Autodesk Inventor part; units mm, degrees
ref_plane "YZ Plane" through (0, 0, 0) normal (1, 0, 0) x (0, 1, 0)
ref_plane "XZ Plane" through (0, 0, 0) normal (0, 1, 0) x (-1, 0, 0)
ref_plane "XY Plane" through (0, 0, 0) normal (0, 0, 1) x (1, 0, 0)
sketch "Boceto1" plane through (0, 0, 0) normal (0, 0, 1) x (1, 0, 0)
  line L0 (0, 0) -> (20, 0)
  line L1 (20, 0) -> (20, 35)
  line L2 (20, 35) -> (0, 35)
  line L3 (0, 35) -> (0, 0)
  line L4 (10, 31) -> (10, 26) construction
  line L5 (8, 31) -> (8, 26)
  line L6 (12, 26) -> (12, 31)
  arc A0 (12, 31) -> (8, 31) centre (10, 31) ccw
  arc A1 (8, 26) -> (12, 26) centre (10, 26) ccw
  line L7 (10, 4) -> (10, 9) construction
  line L8 (12, 4) -> (12, 9)
  line L9 (8, 9) -> (8, 4)
  arc A2 (8, 4) -> (12, 4) centre (10, 4) ccw
  arc A3 (12, 9) -> (8, 9) centre (10, 9) ccw
  point P0 (10, 28.5)
  point P1 (10, 6.5)
  point P2 (10, 33)
  point P3 (10, 2)
  point P4 (10, 11)
  point P5 (10, 24)
  dimension "d0" = 20
  dimension "d1" = 35
  dimension "d2" = 5
  dimension "d3" = 4
  dimension "d4" = 5
  dimension "d5" = 4
  dimension "d6" = 2
  dimension "d7" = 2
  dimension "d8" = 13
extrude "Extrusión1" add sketch "Boceto1" along normal blind 2
sketch "Boceto2" plane through (0, 0, 2) normal (0, 0, 1) x (1, 0, 0)
  line L0 (8, 26) -> (8, 31)
  line L1 (12, 31) -> (12, 26)
  line L2 (8, 21.5) -> (12, 21.5)
  line L3 (12, 21.5) -> (12, 13.5)
  line L4 (12, 13.5) -> (8, 13.5)
  line L5 (8, 13.5) -> (8, 21.5)
  arc A0 (8, 26) -> (12, 26) centre (10, 26) ccw
  arc A1 (12, 9) -> (8, 9) centre (10, 9) ccw
  circle A2 centre (10, 17.5) radius 1.5
  point P0 (0, 0)
  point P1 (10, 21.5)
  point P2 (10, 24)
  point P3 (10, 13.5)
  point P4 (10, 11)
  dimension "d11" = 4
  dimension "d12" = 8
  dimension "d13" = 2.5
  dimension "d15" = 3
extrude "Extrusión2" add sketch "Boceto2" along normal blind 1
sketch "Boceto3" plane through (8, 21.5, 2) normal (0, 1, 0) x (1, 0, 0)
  line L0 (0, -1) -> (0, -6)
  line L1 (4, -1) -> (4, -6)
  arc A0 (0, -6) -> (4, -6) centre (2, -6) ccw
  circle A1 centre (2, -6) radius 1.25
  line L2 (0, -1) -> (4, -1)
  line L3 (0, -1) -> (4, -1)
  point P0 (-8, 2)
  dimension "d18" = 5
  dimension "d19" = 5
  dimension "d20" = 2
  dimension "d21" = 2.5
extrude "Extrusión3" add sketch "Boceto3" against normal blind 1
sketch "Boceto4" plane through (8, 13.5, 2) normal (0, -1, 0) x (1, 0, 0)
  line L0 (0, 0) -> (0, 6)
  line L1 (0, 1) -> (0, 6)
  line L2 (4, 0) -> (4, 1)
  line L3 (4, 1) -> (4, 6)
  line L4 (4, 1) -> (4, 6)
  arc A0 (4, 6) -> (0, 6) centre (2, 6) ccw
  circle A1 centre (2, 6) radius 1.25
  line L5 (0, 1) -> (4, 1)
  line L6 (0, 1) -> (4, 1)
  point P0 (-8, -2)
  dimension "d25" = 2.5
extrude "Extrusión4" add sketch "Boceto4" against normal blind 1
properties part number "soporte_polea"
Geometry check sheet. Reference: the model listing, model coordinates, mm. A direction names the side the tool comes from. Coordinates: 2 decimals unless noted, no trailing zeros. Write each loop counter-clockwise with the first axis right and the second up, starting at its lowest first coordinate (ties: lowest second). Pieces come first, ordered by that corner, then holes. Notation, with made-up numbers: M 26.5,42 L 60.5,42 A25 ccw 60.5,66 Z; hole C 38,-17 d1. An arc over 180 degrees is marked long. One line per item, written item: value. Start each with the question number.
(1) Scan lines: line 1 along Z through (x, y) = (10, 21); line 2 along X through (y, z) = (21, 8); line 3 along Y through (x, z) = (10, 2.65). Record each from-to range of solid material in increasing order. Write a range as [from, to].
(2) Sectioned sample at B-B, the plane y = 28. Enter the section's corners in (x, z), and give its area (3 significant figures).
(3) Sectioned sample at C-C, the plane z = 3.5. Enter the section's corners in (x, y).
(4) Tool access check on faces 1 (the face through (10, 20.5, 6)), 2 (the face through (12, 28, 1)), 3 (the face through (10, 21.5, 5)), 4 (the face through (10, 13.5, 5)). Record the directions out of +Z, -Z, +X, -X, +Y, -Y that give a thin tool (end or side, any length) a straight path to the whole face; none if there is none.
(5) Depth check by flat-ended pin: pin 1 (4 mm diameter, centred on x = 10, y = 17.5, fed in from +Z); pin 2 (5 mm diameter, centred on y = 30, z = 3.5, fed in from -X); pin 3 (3 mm diameter, centred on x = 11, z = 7, fed in from +Y); pin 4 (1.2 mm diameter, centred on x = 9.5, y = 17.5, fed in from +Z). Enter the tip coordinate at first touch or a pass-through.
(6) Release check for a two-part mould opening along X. For faces 5 (the face through (8.89, 16.49, 2.49)), 6 (the face through (10, 21, 10)), 7 (the face through (10, 14.5, 6)) record: released by +X, released by -X, zero draft, split by the parting line, or undercut.
(7) Sectioned sample at D-D, the plane z = 8.5. Enter the section's corners in (x, y).
(8) Sectioned sample at A-A, the plane x = 10. State how many separate pieces and enclosed holes the cut face has, and give its area (3 significant figures).
Filled sheet:
1. line 1: [0, 6.75], [9.25, 10]
1. line 2: [8, 8.75], [11.25, 12]
1. line 3: [13.5, 16], [19, 21.5]
2. outline: M 0,0 L 8,0 L 8,2 L 0,2 Z; M 12,0 L 20,0 L 20,2 L 12,2 Z
2. area: 32.0 mm²
3. outline: M 8,13.5 L 12,13.5 L 12,14.5 L 8,14.5 Z; M 8,20.5 L 12,20.5 L 12,21.5 L 8,21.5 Z
4. face 1: +Z, +X, -X
4. face 2: +Z, -Z
4. face 3: +Z, +X, -X, +Y
4. face 4: +Z, +X, -X, -Y
5. pin 1: z = 3
5. pin 2: x = 0
5. pin 3: y = 21.5
5. pin 4: z = 2
6. face 5: undercut
6. face 6: split by the parting line
6. face 7: zero draft
7. outline: M 8.06,13.5 L 8.85,13.5 L 8.85,14.5 L 8.06,14.5 Z; M 8.06,20.5 L 8.85,20.5 L 8.85,21.5 L 8.06,21.5 Z; M 11.15,13.5 L 11.94,13.5 L 11.94,14.5 L 11.15,14.5 Z; M 11.15,20.5 L 11.94,20.5 L 11.94,21.5 L 11.15,21.5 Z
8. separate pieces: 5
8. enclosed holes: 0
8. area: 48.0 mm²
